Could you check a few things on this model? Use its own coordinates, in mm. A direction names the side the tool comes from. Round coordinates to 2 decimals unless told otherwise and drop trailing zeros. Loops run counter-clockwise (first coordinate to the right, second up) from the corner with the lowest first, then second, coordinate; pieces in that order, holes last. Notation, with made-up numbers: (65.25, 11.5) -> (94.25, 11.5) arc R26 cw to (94.25, 48.5) -> close; hole circle Ø6 at (41, 3). An arc over 180 degrees is marked (long way). Put each result on its own line as item: value. Start each with the question number.
1. Imagine slicing it at C-C, the plane y = 25. Please give me the cut outline in (x, z).
2. Imagine slicing it at A-A, the plane x = -34. Please give me the cut outline in (y, z).
3. I need wall thicknesses on line 1 (X direction, y = 27, z = 12); line 2 (Z direction, x = -40.5, y = 21); line 3 (X direction, y = 20, z = 26.5). Which ranges of each line are inside material? Lowest first, please. Write a range as [from, to].
4. If we mould it in two halves opening along Z, with no side actions, what happens to faces 1 (the flat face through (-55.909, 7, 25)), 2 (the flat face through (-33, 12, 45)), 3 (the flat face through (-29, 7, 50)), 4 (the flat face through (-29, 13, 0))? For each: pulls with the +Z half, pulls with the -Z half, needs draft (parallel to the pull), parting line crosses it, or undercut.
5. Imagine slicing it at D-D, the plane y = 20. Please give me the cut outline in (x, z).
6. I'm going to push flat-ended pins straight in: P1, Ø11.5, axis at x = -27, z = 32.5, coming from the +Y side; P2, Ø1.1, axis at y = -5, z = 2, coming from the +X side; P3, Ø4.5, axis at x = 8, z = 26, coming from the -Y side. Where does each tip first touch, or does it pass through?
7. Which directions (+Z, -Z, +X, -X, +Y, -Y) give clear straight access to the entire face, cutting with the end or side of a thin tool? Please do faces 5 (the flat face through (-8.066, 1.538, 24.65)), 6 (the flat face through (9, 11.818, 25)), 7 (the flat face through (-13.909, 12, 25)), 8 (the flat face through (-31.566, -5, 3)).
8. Imagine slicing it at B-B, the plane z = 6. Please give me the cut outline in (x, y), and give its area (3 significant figures).
```python
from build123d import *

# Parameters (mm, degrees)
BOSS_EXTRUDE1_DEPTH = 50
SKETCH2_W           = 38.381895626
SKETCH2_H           = 40
CUT_EXTRUDE2_DEPTH  = 41
SKETCH4_W           = 6.790896345
SKETCH4_H           = 3.798015254
CUT_EXTRUDE3_DEPTH  = 5


with BuildPart() as part:
    # Sketch1 → Boss-Extrude1 (new body)
    with BuildSketch(Plane.XY):
        Polygon((-55.909090909, 31.818181818), (-55.909090909, -18.181818182), (-15.909090909, -18.181818182), (0, 21.818181818), (5, 21.818181818), (5, 11.818181818), (14.090909091, 11.818181818), (14.090909091, 31.818181818), align=None)
    extrude(amount=BOSS_EXTRUDE1_DEPTH)

    # Sketch2 → Cut-Extrude2 (cut)
    with BuildSketch(Plane(origin=(0, 31.818181818, 0), x_dir=(1, 0, 0), z_dir=(0, 1, 0))):
        with Locations((-33.100038722, -25)):
            Rectangle(SKETCH2_W, SKETCH2_H)
    extrude(amount=-CUT_EXTRUDE2_DEPTH, mode=Mode.SUBTRACT)

    # Sketch4 → Cut-Extrude3 (cut)
    with BuildSketch(Plane.XY.offset(5)):
        with Locations((-34.961451434, -5.442472673)):
            Rectangle(SKETCH4_W, SKETCH4_H)
    extrude(amount=-CUT_EXTRUDE3_DEPTH, mode=Mode.SUBTRACT)


solid = part.part
```
Entries:
1. outline: (-55.91, 0) -> (14.09, 0) -> (14.09, 50) -> (-55.91, 50) -> close; hole (-52.29, 5) -> (-13.91, 5) -> (-13.91, 45) -> (-52.29, 45) -> close
2. outline: (-18.18, 0) -> (-7.34, 0) -> (-7.34, 5) -> (-9.18, 5) -> (-9.18, 45) -> (31.82, 45) -> (31.82, 50) -> (-18.18, 50) -> close; (-3.54, 0) -> (31.82, 0) -> (31.82, 5) -> (-3.54, 5) -> close
3. line 1: [-55.91, -52.29], [-13.91, 14.09]
3. line 2: [0, 5], [45, 50]
3. line 3: [-55.91, -52.29], [-13.91, -0.72], [5, 14.09]
4. face 1: needs draft
4. face 2: undercut
4. face 3: pulls with the +Z half
4. face 4: pulls with the -Z half
5. outline: (-55.91, 0) -> (-0.72, 0) -> (-0.72, 50) -> (-55.91, 50) -> close; (5, 0) -> (14.09, 0) -> (14.09, 50) -> (5, 50) -> close; hole (-52.29, 5) -> (-13.91, 5) -> (-13.91, 45) -> (-52.29, 45) -> close
6. P1: y = -9.18
6. P2: x = -10.45
6. P3: y = 11.82
7. face 5: +Z, -Z, -Y
7. face 6: +Z, -Z, +X, -Y
7. face 7: +Y
7. face 8: -Z
8. outline: (-55.91, -18.18) -> (-15.91, -18.18) -> (0, 21.82) -> (5, 21.82) -> (5, 11.82) -> (14.09, 11.82) -> (14.09, 31.82) -> (-13.91, 31.82) -> (-13.91, -9.18) -> (-52.29, -9.18) -> (-52.29, 31.82) -> (-55.91, 31.82) -> close
8. area: 1,140 mm^2
